Part model, mm, in its own coordinate system. A direction names the side the tool comes from. Coordinates: 2 decimals unless noted, no trailing zeros. Order: outer loops, then holes, each group sorted by start corner. A loop starts at its lowest first (then second) coordinate and runs counter-clockwise, first axis right, second up.
from build123d import *

# Parameters (mm, degrees)
BALAYAGE1_PROFILE_R = 1.5


with BuildPart() as part:
    # Balayage1: sweep along a curve in space
    with BuildLine() as balayage1_path:
        Line((0, 0, 0), (0, 15, 0))
        ThreePointArc((0, 15, 0), (0, 22.071067812, -2.928932188), (0, 25, -10))
        Line((0, 25, -10), (0, 25, -15))
        ThreePointArc((0, 25, -15), (2.928932188, 25, -22.071067812), (10, 25, -25))
        Line((10, 25, -25), (40, 25, -25))
    # Balayage1 profile (on start of the path) → Balayage1 (sweep)
    with BuildSketch(Plane.ZX):
        Circle(BALAYAGE1_PROFILE_R)
    sweep(path=balayage1_path.line)


solid = part.part
Q1. Wall check: line 1 along X through (y, z) = (23.5, -5); line 2 along Z through (x, y) = (1, 10). Give the ranges that are in metal, low to high.
Results list:
line 1: x = -1.49 to 1.49
line 2: z = -1.12 to 1.12
Q2. Which spindle directions (+Z, -Z, +X, -X, +Y, -Y) get a long thin tool onto all of the face, cutting with end or side? Do faces 4 (the face through (25.21, 23.89, -23.99)), 5 (the face through (0, 0, 0)). Say none if no direction does.
Results list:
face 4: +X
face 5: +Z, -Z, +X, -X, -Y
Q3. Cut at B-B on z = -10.5. Write the cut outline in (x, y).
Results list:
outline: circle Ø3 at (0, 25)
Q4. Mould opens along Z. For faces 1 (the face through (40, 25, -25)), 2 (the face through (0.07, 23.5, -12.54)), 3 (the face through (0.07, 7.6, -1.5)) say: pulls with the +Z half, pulls with the -Z half, needs draft (parallel to the pull), parting line crosses it, or undercut.
Results list:
face 1: needs draft
face 2: undercut
face 3: parting line crosses it
Q5. Cut at A-A on y = 11. Write the cut outline in (x, z).
Results list:
outline: circle Ø3 at (0, 0)
Q6. Pin check, flat tips, straight feed: pin 1 Ø4 at (y, z) = (10, -3) entering from +X; pin 2 Ø10 at (x, y) = (12.5, 20.5) entering from -Z. Stop position of each tip, or through.
Results list:
pin 1: stops at x = 1.12
pin 2: stops at z = -26.5
